The figure shows three views and two pictorial views of one solid part (mm, origin at its lowest corner). Answer the questions. Coordinates: 2 decimals unless noted, no trailing zeros. Write each loop counter-clockwise with the first axis right and the second up, starting at its lowest first coordinate (ties: lowest second). Pieces come first, ordered by that corner, then holes. Notation, with made-up numbers: (16.25, 60) - (27.25, 60) arc R27 cw to (27.25, 94) - close; hole circle Ø3 at (-21.75, 2.25). An arc over 180 degrees is marked (long way). Use a Markdown table: item, result. Add a question column.
(1) The part is cut by section D-D, the plane z = 17.5. Give the vertices of the cut face in (x, y), then the cut area to 3 significant figures.
(2) Given pin 1 Ø1.2 at (x, y) = (2.5, 5.5) entering from -Z, flat-ended and moving along its own axis, determine where the tip first touches the part or whether it passes through.
(3) The part is cut by section B-B, the plane x = 1.7. Give the vertices of the cut face in (y, z), then the cut area to 3 significant figures.
(4) The part is cut by section A-A, the plane y = 112. Give the vertices of the cut face in (x, z), then the cut area to 3 significant figures.
(5) Find the intervals of material crossed by line 1 (Z direction, x = 3.25, y = 92); line 2 (Y direction, x = 2.1, z = 2.5); line 3 (Y direction, x = 1.4, z = 9), in increasing order. Write a range as from..to.
(6) The part is cut by section C-C, the plane y = 29. Give the vertices of the cut face in (x, z), then the cut area to 3 significant figures.
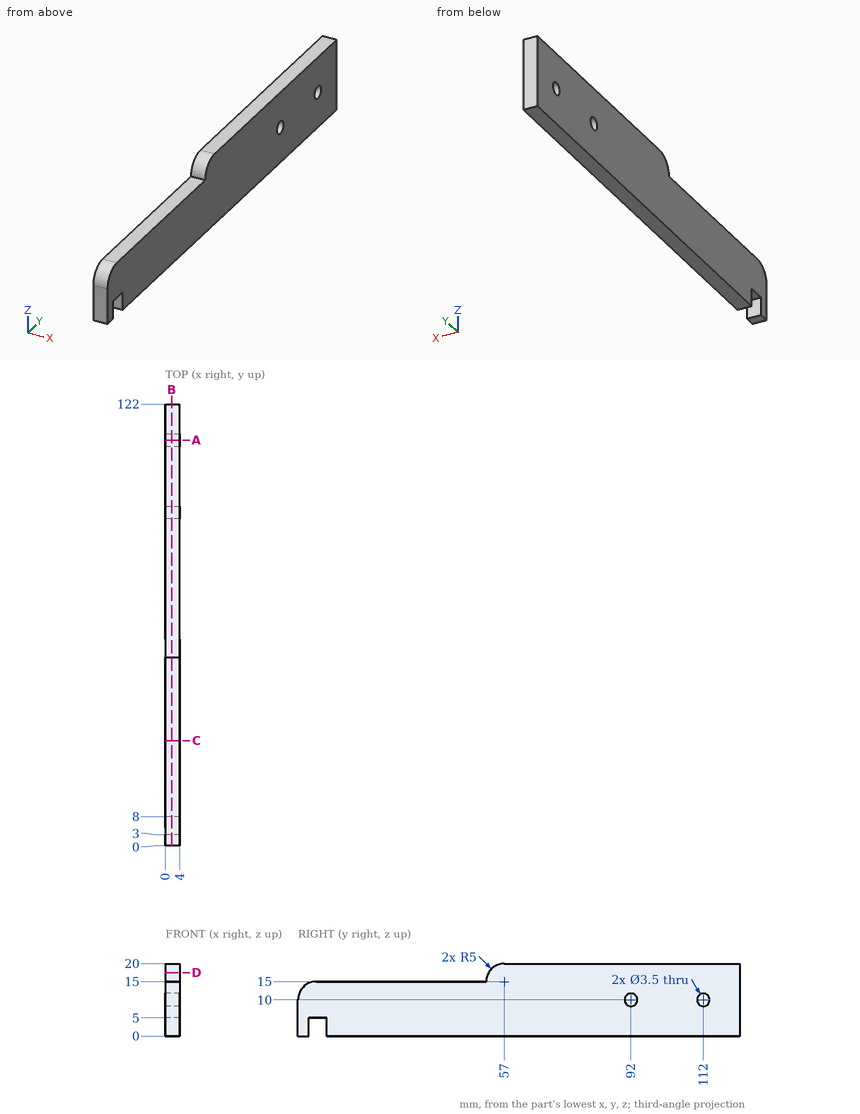
Model answer:
| question | item | result |
|---|---|---|
| 1 | outline | (0, 52.67) - (4, 52.67) - (4, 122) - (0, 122) - close |
| 1 | area | 277 mm^2 |
| 2 | pin 1 | z = 5 |
| 3 | outline | (0, 0) - (3, 0) - (3, 5) - (8, 5) - (8, 0) - (122, 0) - (122, 20) - (57, 20) arc R5 ccw to (52, 15) - (5, 15) arc R5 ccw to (0, 10) - close; hole circle Ø3.5 at (92, 10); hole circle Ø3.5 at (112, 10) |
| 3 | area | 2,130 mm^2 |
| 4 | outline | (0, 0) - (4, 0) - (4, 8.25) - (0, 8.25) - close; (0, 11.75) - (4, 11.75) - (4, 20) - (0, 20) - close |
| 4 | area | 66.0 mm^2 |
| 5 | line 1 | 0..8.25, 11.75..20 |
| 5 | line 2 | 0..3, 8..122 |
| 5 | line 3 | 0..90.56, 93.44..110.56, 113.44..122 |
| 6 | outline | (0, 0) - (4, 0) - (4, 15) - (0, 15) - close |
| 6 | area | 60.0 mm^2 |
